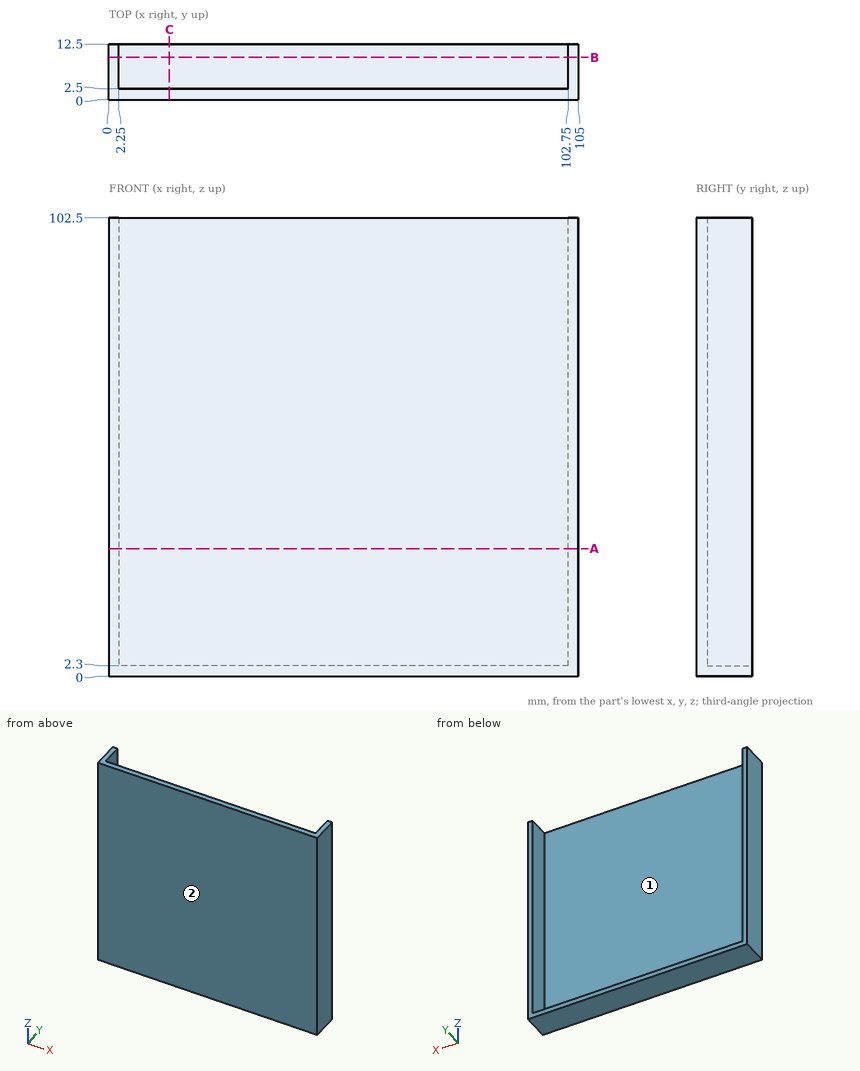
Drawing for the job (mm, zero at the part's lowest x, y, z). A direction names the side the tool comes from. Round coordinates to 2 decimals unless told otherwise and drop trailing zeros. Loops run counter-clockwise (first coordinate to the right, second up) from the corner with the lowest first, then second, coordinate; pieces in that order, holes last. Notation, with made-up numbers: (-37.5, 54) -> (-32.5, 54) arc R28 ccw to (-32.5, 76) -> close; hole circle Ø7 at (89, 3). An arc over 180 degrees is marked (long way). Answer in a Markdown table with one row per item.
Item 1: Drill centre lines: L1, parallel to X at y = 4, z = 74; L2, parallel to Y at x = 31.5, z = 10; L3, parallel to Z at x = 52, y = 6. Where is each one in solid material? Low to high. Write a range as [from, to].
Answers below:
| item | result |
|---|---|
| L1 | x = [0, 2.25], [102.75, 105] |
| L2 | y = [0, 2.5] |
| L3 | z = [0, 2.3] |
Item 2: Saw through at A-A (z = 28.5). Write the cut outline in (x, y), and give its area (4 significant figures).
Answers below:
| item | result |
|---|---|
| outline | (0, 0) -> (105, 0) -> (105, 12.5) -> (102.75, 12.5) -> (102.75, 2.5) -> (2.25, 2.5) -> (2.25, 12.5) -> (0, 12.5) -> close |
| area | 307.5 mm² |
Item 3: Saw through at C-C (x = 13.5). Write the cut outline in (y, z).
Answers below:
| item | result |
|---|---|
| outline | (0, 0) -> (12.5, 0) -> (12.5, 2.3) -> (2.5, 2.3) -> (2.5, 102.5) -> (0, 102.5) -> close |
Item 4: Saw through at B-B (y = 9.5). Write the cut outline in (x, z), and give its area (3 significant figures).
Answers below:
| item | result |
|---|---|
| outline | (0, 0) -> (105, 0) -> (105, 102.5) -> (102.75, 102.5) -> (102.75, 2.3) -> (2.25, 2.3) -> (2.25, 102.5) -> (0, 102.5) -> close |
| area | 692 mm² |
Item 5: Which spindle directions (+Z, -Z, +X, -X, +Y, -Y) get a long thin tool onto all of the face, cutting with end or side? Do the marked faces 1 and 2. Say none if no direction does.
Answers below:
| item | result |
|---|---|
| face 1 | +Z, +Y |
| face 2 | +Z, -Z, +X, -X, -Y |
Item 6: Pin check, flat tips, straight feed: pin 1 (6 mm diameter, centred on x = 43.5, y = 6, fed in from +Z); pin 2 (4 mm diameter, centred on x = 33, z = 73, fed in from +Y). Stop position of each tip, or through.
Answers below:
| item | result |
|---|---|
| pin 1 | stops at z = 2.3 |
| pin 2 | stops at y = 2.5 |
